The listing builds one solid part. Answer for the finished solid, in the listing's coordinates (mm). Face numbers are marked on the shaded views. A direction names the side the tool comes from. Give positions to 0.01 mm unless a question says otherwise; leave off trailing zeros. Order: outer loops, then holes, each group sorted by start corner. A loop starts at its lowest first (then second) coordinate and runs counter-clockwise, first axis right, second up. Notation, with made-up numbers: (20, 4) -> (61, 4) arc R17 ccw to (61, 10) -> close; hole circle Ø2 at (-5.75, 59). An arc over 180 degrees is marked (long way). Answer as a JSON object with one key per item and string values. Group by question number.
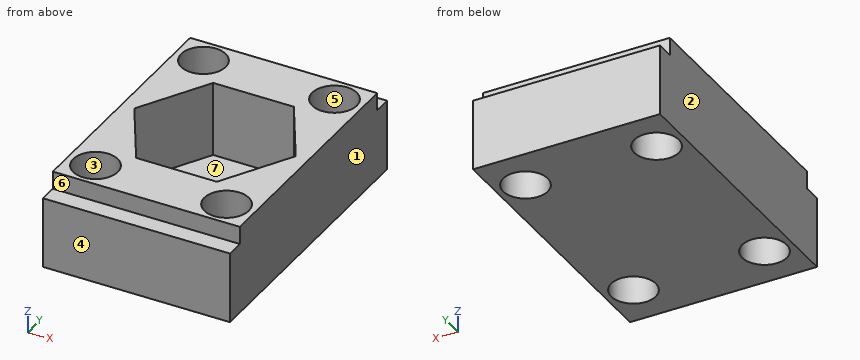
```python
from build123d import *

# Parameters (mm, degrees)
BOX_W           = 21
BOX_H           = 32
BOX_DEPTH       = 10
POCKET_DEPTH    = 8.4
SKETCH002_W     = 21
SKETCH002_H     = 2
POCKET001_DEPTH = 2
SKETCH001_R     = 2.5
POCKET002_DEPTH = 10.001


with BuildPart() as part:
    # Box → Box (new body)
    with BuildSketch(Plane.XY):
        with Locations((10.5, 16)):
            Rectangle(BOX_W, BOX_H)
    extrude(amount=BOX_DEPTH)

    # Sketch → Pocket (cut)
    with BuildSketch(Plane.XY.offset(10)):
        Polygon((1.435601, 16), (5.9678, 23.850001), (15.0322, 23.850001), (19.564399, 16), (15.0322, 8.149999), (5.9678, 8.149999), align=None)
    extrude(amount=-POCKET_DEPTH, mode=Mode.SUBTRACT)

    # Sketch002 → Pocket001 (cut)
    with BuildSketch(Plane.XY.offset(10)):
        with Locations((10.5, 31)):
            Rectangle(SKETCH002_W, SKETCH002_H)
        with Locations((10.5, 1)):
            Rectangle(SKETCH002_W, SKETCH002_H)
    extrude(amount=-POCKET001_DEPTH, mode=Mode.SUBTRACT)

    # Sketch001 → Pocket002 (cut, through all)
    with BuildSketch(Plane.XY.offset(10)):
        with Locations((3.140495, 27)):
            Circle(SKETCH001_R)
        with Locations((17.859505, 27)):
            Circle(SKETCH001_R)
        with Locations((3.140495, 5)):
            Circle(SKETCH001_R)
        with Locations((17.859505, 5)):
            Circle(SKETCH001_R)
    extrude(amount=-POCKET002_DEPTH, mode=Mode.SUBTRACT)


solid = part.part
```
(1) A cutting plane is placed at B-B (y = 27). Determine the outline of the cut face in (x, z).
(2) For a pull along X with two mould halves and no side action, classify the marked faces 1, 2, 3 and 4 as +X half, -X half, draft (parallel to the pull), parting line (faces both ways), or undercut.
(3) Which of the six approach directions +Z, -Z, +X, -X, +Y, -Y give full straight-line access (tool end or side, diameter ignored) to the marked faces 5, 6 and 7?
(4) A cutting plane is placed at A-A (z = 1). Determine the outline of the cut face in (x, y).
(5) A cutting plane is placed at D-D (z = 6). Determine the outline of the cut face in (x, y), and give its area (3 significant figures).
(6) Find the intervals of material crossed by line 1 along Y through (x, z) = (3, 0.5); line 2 along Y through (x, z) = (14.75, 3.5); line 3 along Y through (x, z) = (15, 9.75), in increasing order. Write a range as [from, to].
(7) A cutting plane is placed at C-C (x = 14). Determine the outline of the cut face in (y, z).
(8) Flat-ended cylindrical pins translate along their axes: pin 1 Ø1 at (x, y) = (15, 31.5) entering from +Z; pin 2 Ø1 at (x, z) = (7, 9) entering from +Y. Find the tip coordinate at first contact, or state that the pin passes through.
Check sheet entries:
{
 "1": {"outline": "(0, 0) -> (0.64, 0) -> (0.64, 10) -> (0, 10) -> close; (5.64, 0) -> (15.36, 0) -> (15.36, 10) -> (5.64, 10) -> close; (20.36, 0) -> (21, 0) -> (21, 10) -> (20.36, 10) -> close"},
 "2": {"face 1": "+X half", "face 2": "-X half", "face 3": "undercut", "face 4": "draft"},
 "3": {"face 5": "+Z, -Z", "face 6": "+Z, +X, -X, -Y", "face 7": "+Z"},
 "4": {"outline": "(0, 0) -> (21, 0) -> (21, 32) -> (0, 32) -> close; hole circle Ø5 at (3.14, 5); hole circle Ø5 at (3.14, 27); hole circle Ø5 at (17.86, 5); hole circle Ø5 at (17.86, 27)"},
 "5": {"outline": "(0, 0) -> (21, 0) -> (21, 32) -> (0, 32) -> close; hole circle Ø5 at (3.14, 5); hole circle Ø5 at (3.14, 27); hole (1.44, 16) -> (5.97, 8.15) -> (15.03, 8.15) -> (19.56, 16) -> (15.03, 23.85) -> (5.97, 23.85) -> close; hole circle Ø5 at (17.86, 5); hole circle Ø5 at (17.86, 27)", "area": "380 mm2"},
 "6": {"line 1": "y = [0, 2.5], [7.5, 24.5], [29.5, 32]", "line 2": "y = [0, 8.15], [23.85, 32]", "line 3": "y = [2, 8.15], [23.85, 30]"},
 "7": {"outline": "(0, 0) -> (32, 0) -> (32, 8) -> (30, 8) -> (30, 10) -> (23.85, 10) -> (23.85, 1.6) -> (8.15, 1.6) -> (8.15, 10) -> (2, 10) -> (2, 8) -> (0, 8) -> close"},
 "8": {"pin 1": "stops at z = 8", "pin 2": "stops at y = 30"}
}
